```python
from build123d import *

# Parameters (mm, degrees)
SKETCH1_R           = 8.255
BOSS_EXTRUDE1_DEPTH = 78.7908
SKETCH3_W           = 28.144543877
SKETCH3_H           = 0.9906
SKETCH4_W           = 12.873525148
SKETCH4_H           = 0.9906
SKETCH5_W           = 18.510298187
SKETCH5_H           = 0.9906
SKETCH6_W           = 13.338836726
SKETCH6_H           = 0.9906
CUT_EXTRUDE2_DEPTH  = 2.7432
CUT_EXTRUDE3_DEPTH  = 2.7432


with BuildPart() as part:
    # Sketch1 → Boss-Extrude1 (new body)
    with BuildSketch(Plane(origin=(0, 0, 0), x_dir=(1, 0, 0), z_dir=(0, 1, 0))):
        Circle(SKETCH1_R)
    extrude(amount=BOSS_EXTRUDE1_DEPTH)

    # Sketch3 → Cut-Revolve1 (revolve, cut)
    with BuildSketch(Plane(origin=(0, 0, 0), x_dir=(0, 0, -1), z_dir=(1, 0, 0))):
        with Locations((-21.857371939, 16.3703)):
            Rectangle(SKETCH3_W, SKETCH3_H)
    revolve(axis=Axis((0, 29.927318778, 0), (0, -1, 0)), mode=Mode.SUBTRACT)

    # Sketch4 → Cut-Revolve2 (revolve, cut)
    with BuildSketch(Plane(origin=(0, 0, 0), x_dir=(0, 0, -1), z_dir=(1, 0, 0))):
        with Locations((-14.221862574, 30.0609)):
            Rectangle(SKETCH4_W, SKETCH4_H)
    revolve(axis=Axis((0, 33.790657772, 0), (0, -1, 0)), mode=Mode.SUBTRACT)

    # Sketch5 → Cut-Revolve3 (revolve, cut)
    with BuildSketch(Plane(origin=(0, 0, 0), x_dir=(0, 0, -1), z_dir=(1, 0, 0))):
        with Locations((-17.040249094, 56.0705)):
            Rectangle(SKETCH5_W, SKETCH5_H)
    revolve(axis=Axis((0, 60.607773061, 0), (0, -1, 0)), mode=Mode.SUBTRACT)

    # Sketch6 → Cut-Revolve4 (revolve, cut)
    with BuildSketch(Plane(origin=(0, 0, 0), x_dir=(0, 0, -1), z_dir=(1, 0, 0))):
        with Locations((-14.454518363, 76.1111)):
            Rectangle(SKETCH6_W, SKETCH6_H)
    revolve(axis=Axis((0, 77.155375287, 0), (0, -1, 0)), mode=Mode.SUBTRACT)

    # Sketch7 → Cut-Extrude2 (cut)
    with BuildSketch(Plane(origin=(8.2804, 0, 0), x_dir=(0, 0, -1), z_dir=(1, 0, 0))):
        with BuildLine():
            Line((2.3876, 75.6158), (2.3876, 56.5658))
            ThreePointArc((2.3876, 56.5658), (0, 54.1782), (-2.3876, 56.5658))
            Line((-2.3876, 56.5658), (-2.3876, 75.6158))
            ThreePointArc((-2.3876, 75.6158), (0, 78.0034), (2.3876, 75.6158))
        make_face()
    extrude(amount=-CUT_EXTRUDE2_DEPTH, mode=Mode.SUBTRACT)

    # Sketch8 → Cut-Extrude3 (cut)
    with BuildSketch(Plane(origin=(8.2804, 0, 0), x_dir=(0, 0, -1), z_dir=(1, 0, 0))):
        with BuildLine():
            Line((2.3876, 29.5656), (2.3876, 16.8656))
            ThreePointArc((2.3876, 16.8656), (0, 14.478), (-2.3876, 16.8656))
            Line((-2.3876, 16.8656), (-2.3876, 29.5656))
            ThreePointArc((-2.3876, 29.5656), (0, 31.9532), (2.3876, 29.5656))
        make_face()
    extrude(amount=-CUT_EXTRUDE3_DEPTH, mode=Mode.SUBTRACT)


solid = part.part
```
Here's how the part is built. I have some questions about the finished solid (model axes, mm). A direction names the side the tool comes from. Coordinates: 2 decimals unless noted, no trailing zeros. Loops run counter-clockwise (first coordinate to the right, second up) from the corner with the lowest first, then second, coordinate; pieces in that order, holes last. Notation, with made-up numbers: (-6.5, 26) - (27.5, 26) arc R3 ccw to (27.5, 30) - close; hole circle Ø5 at (32, 5). An arc over 180 degrees is marked (long way). Return JSON: item names as keys, results as strings. Group by question number.
Item 1: On a 3-axis mill with a long thin cutter (end or side, diameter ignored), from which of +Z, -Z, +X, -X, +Y, -Y can I reach the whole of each face in a straight line? I mean faces 1 (the face through (6.9, 78, 0.1)), 2 (the face through (7.874, 42.891, -2.48)), 3 (the face through (-8, 29.566, 0)). Say none if no direction works.
Item 2: I need wall thicknesses on line 1 (Y direction, x = -6.75, z = -4) (3 decimals); line 2 (Y direction, x = 7.5, z = 2); line 3 (Y direction, x = 7, z = -1). Which ranges of each line are inside material? Lowest first, please. Write a range as from..to.
Item 3: If we section it at C-C on y = 24: Write out the boundary of the cut face in (x, z) (3 decimals), and give its area (3 significant figures).
Item 4: Will these pins go through, and if not, where does the flat tip stop? P1, Ø2, axis at x = -6, y = 34, coming from the -Z side; P2, Ø1.2, axis at x = 6.5, y = 23, coming from the +Z side; P3, Ø1.4, axis at y = 25, z = -1, coming from the +X side.
Item 5: If we section it at A-A on z = 0: Write out the boundary of the cut face in (x, y) (3 decimals).
Item 6: We'd pull the mould along Y, two halves only. Please class faces 4 (the face through (0, 0, 0)), 5 (the face through (7.874, 7.826, -2.48)), 6 (the face through (5.537, 23, 0)): +Y half, -Y half, draft (parallel to the pull), parting line (faces both ways), or undercut.
Item 7: If we section it at B-B on y = 7: Write out the boundary of the cut face in (x, z) (3 decimals).
Calculated:
{
 "1": {"face 1": "+X", "face 2": "+Y, -Y", "face 3": "none"},
 "2": {"line 1": "y = 0..15.875, 16.866..29.566, 30.556..55.575, 56.566..75.616, 76.606..78.791", "line 2": "y = 0..15.56, 30.87..55.26, 76.92..78.79", "line 3": "y = 0..14.7, 31.73..54.4, 77.78..78.79"},
 "3": {"outline": "(5.537, -2.388) - (5.537, 2.388) - (7.902, 2.388) arc R8.255 ccw (long way) to (7.902, -2.388) - close", "area": "202 mm^2"},
 "4": {"P1": "stops at z = -6.57", "P2": "stops at z = 5.77", "P3": "stops at x = 5.54"},
 "5": {"outline": "(-8.255, 0) - (8.255, 0) - (8.255, 14.478) - (5.537, 14.478) - (5.537, 31.953) - (8.255, 31.953) - (8.255, 54.178) - (5.537, 54.178) - (5.537, 78.003) - (8.255, 78.003) - (8.255, 78.791) - (-8.255, 78.791) - (-8.255, 76.606) - (-7.785, 76.606) - (-7.785, 75.616) - (-8.255, 75.616) - (-8.255, 56.566) - (-7.785, 56.566) - (-7.785, 55.575) - (-8.255, 55.575) - (-8.255, 30.556) - (-7.785, 30.556) - (-7.785, 29.566) - (-8.255, 29.566) - (-8.255, 16.866) - (-7.785, 16.866) - (-7.785, 15.875) - (-8.255, 15.875) - close"},
 "6": {"face 4": "-Y half", "face 5": "draft", "face 6": "undercut"},
 "7": {"outline": "circle Ø16.51 at (0, 0)"}
}
